```python
from build123d import *

# Parameters (mm, degrees)
SKETCH1_R           = 4.699
BOSS_EXTRUDE1_DEPTH = 2.54


with BuildPart() as part:
    # Sketch1 → Boss-Extrude1 (new body)
    with BuildSketch(Plane.XY):
        Polygon((0, 234.635149399), (-203.2, -117.317574699), (203.2, -117.317574699), align=None)
        with Locations((0, -82.55)):
            Circle(SKETCH1_R, mode=Mode.SUBTRACT)
        with Locations((-71.490397082, 41.275)):
            Circle(SKETCH1_R, mode=Mode.SUBTRACT)
        with Locations((71.490397082, 41.275)):
            Circle(SKETCH1_R, mode=Mode.SUBTRACT)
        with BuildLine():
            Line((-2.54, 72.188105961), (-2.54, 197.994436105))
            Line((-2.54, 197.994436105), (2.54, 197.994436105))
            Line((2.54, 197.994436105), (2.54, 72.188105961))
            ThreePointArc((2.54, 72.188105961), (6.987296904, 57.830382152), (18.771829368, 48.500458394))
            ThreePointArc((18.771829368, 48.500458394), (45.038950162, 26.00325), (51.388543748, -7.993348088))
            ThreePointArc((51.388543748, -7.993348088), (53.576228506, -22.864014453), (63.786733613, -33.894348455))
            Line((63.786733613, -33.894348455), (172.738211475, -96.797513527))
            Line((172.738211475, -96.797513527), (170.198211475, -101.196922578))
            Line((170.198211475, -101.196922578), (61.246733613, -38.293757506))
            ThreePointArc((61.246733613, -38.293757506), (46.588931602, -34.966367699), (32.61671438, -40.507110305))
            ThreePointArc((32.61671438, -40.507110305), (0, -52.0065), (-32.61671438, -40.507110305))
            ThreePointArc((-32.61671438, -40.507110305), (-46.588931602, -34.966367699), (-61.246733613, -38.293757506))
            Line((-61.246733613, -38.293757506), (-170.198211475, -101.196922578))
            Line((-170.198211475, -101.196922578), (-172.738211475, -96.797513527))
            Line((-172.738211475, -96.797513527), (-63.786733613, -33.894348455))
            ThreePointArc((-63.786733613, -33.894348455), (-53.576228506, -22.864014453), (-51.388543748, -7.993348088))
            ThreePointArc((-51.388543748, -7.993348088), (-45.038950162, 26.00325), (-18.771829368, 48.500458394))
            ThreePointArc((-18.771829368, 48.500458394), (-6.987296904, 57.830382152), (-2.54, 72.188105961))
        make_face(mode=Mode.SUBTRACT)
    extrude(amount=BOSS_EXTRUDE1_DEPTH)


solid = part.part
```
The model under review builds one solid part; all positions refer to its coordinate system, in mm. A direction names the side the tool comes from. Round coordinates to 2 decimals unless told otherwise and drop trailing zeros. Loops run counter-clockwise (first coordinate to the right, second up) from the corner with the lowest first, then second, coordinate; pieces in that order, holes last.
Item 1: For faces 1 (the face through (0.494, -52.004, 1.252)), 2 (the face through (-48, 22, 2.54)), list the 3-axis set-ups (+Z, -Z, +X, -X, +Y, -Y) from which the entire face can be reached by the end or side of a thin tool; tool diameter is ignored.
Determined:
face 1: +Z, -Z
face 2: +Z, +X, -X, +Y, -Y
Item 2: Mouldability with a two-part tool opening along X and no side actions: class faces 3 (the face through (-48, 22, 0)), 4 (the face through (103.02, 56.2, 1.25)), 5 (the face through (-53.67, -23.06, 1.25)) as released by +X, released by -X, zero draft, split by the parting line, or undercut.
Determined:
face 3: zero draft
face 4: released by +X
face 5: undercut
Item 3: Clearance check with flat-ended pins moving along their axes: pin 1 Ø0.8 at (y, z) = (165, 1) entering from +X; pin 2 Ø0.8 at (y, z) = (155, 1.5) entering from -X; pin 3 Ø1 at (y, z) = (19, 2) entering from -X. State where each tip first meets the part, or that it passes through.
Determined:
pin 1: stops at x = 40.43
pin 2: stops at x = -46.21
pin 3: stops at x = -124.79
Item 4: Take a section at A-A (y = 112). Write out the cut boundary in (x, z), then the cut area to 3 significant figures.
Determined:
outline: (-70.8, 0) - (-2.54, 0) - (-2.54, 2.54) - (-70.8, 2.54) - close; (2.54, 0) - (70.8, 0) - (70.8, 2.54) - (2.54, 2.54) - close
area: 347 mm2
Item 5: Take a section at D-D (z = 0.6). Give the number of separate pieces and of enclosed holes in the cut face, then the cut area to 3 significant figures.
Determined:
separate pieces: 1
enclosed holes: 4
area: 60,200 mm2
Item 6: Take a section at C-C (y = -82.55). Write out the cut boundary in (x, z).
Determined:
outline: (-183.13, 0) - (-148.06, 0) - (-148.06, 2.54) - (-183.13, 2.54) - close; (-137.9, 0) - (-4.7, 0) - (-4.7, 2.54) - (-137.9, 2.54) - close; (4.7, 0) - (137.9, 0) - (137.9, 2.54) - (4.7, 2.54) - close; (148.06, 0) - (183.13, 0) - (183.13, 2.54) - (148.06, 2.54) - close
Item 7: Take a section at B-B (x = 133). Write out the cut boundary in (y, z), then the cut area to 3 significant figures.
Determined:
outline: (-117.32, 0) - (-79.72, 0) - (-79.72, 2.54) - (-117.32, 2.54) - close; (-73.85, 0) - (4.27, 0) - (4.27, 2.54) - (-73.85, 2.54) - close
area: 294 mm2
Item 8: For line 1 (Y direction, x = 0, z = 1.3); line 2 (X direction, y = -38, z = 0.55); line 3 (X direction, y = -86, z = 1.8), list the stretches that pass through material, from the lowest coordinate up.
Determined:
line 1: y = -117.32 to -87.25, -77.85 to -52.01, 197.99 to 234.64
line 2: x = -157.41 to -70.9, -60.72 to -36.37, 36.37 to 60.72, 70.9 to 157.41
line 3: x = -185.12 to -154.04, -143.88 to -3.19, 3.19 to 143.88, 154.04 to 185.12
